Design review of the part built by this model. Coordinates are the model's own, in mm. Face numbers are marked on the shaded views. A direction names the side the tool comes from. Round coordinates to 2 decimals unless told otherwise and drop trailing zeros. Loops run counter-clockwise (first coordinate to the right, second up) from the corner with the lowest first, then second, coordinate; pieces in that order, holes last. Notation, with made-up numbers: (49, 31.5) - (55, 31.5) arc R26 cw to (55, 57.5) - close; hole circle Ø6 at (-40, 77). An arc over 180 degrees is marked (long way). Return JSON: item names as keys, results as strings. Group by question number.
(1) We need section C-C, the plane x = 25.5. Write out the cut boundary in (y, z), and give its area (3 significant figures).
(2) For the marked faces 1 and 2, list the 3-axis set-ups (+Z, -Z, +X, -X, +Y, -Y) from which the entire face can be reached by the end or side of a thin tool; tool diameter is ignored.
(3) The part is to be moulded in two halves that separate along X. For the marked faces 3, 4 and 5, say which applies: pulls with the +X half, pulls with the -X half, needs draft (parallel to the pull), parting line crosses it, or undercut.
(4) Clearance check with flat-ended pins moving along their axes: pin 1 (3.5 mm diameter, centred on x = 16, z = 26, fed in from -Y); pin 2 (1.5 mm diameter, centred on x = 14, y = 4.5, fed in from +Z); pin 3 (2.5 mm diameter, centred on x = 25.5, y = 6.5, fed in from -Z). State where each tip first meets the part, or that it passes through.
(5) We need section D-D, the plane z = 26. Give the number of separate pieces and of enclosed holes in the cut face, and give its area (3 significant figures).
(6) We need section A-A, the plane z = 51.5. Write out the cut boundary in (x, y).
(7) Wall thickness on L1, parallel to Z at x = 29.75, y = 6.5; L2, parallel to Y at x = 1.7, z = 26; L3, parallel to X at y = 6.5, z = 62.4: over which ranges is each line inside the solid? List them lowest first. Write a range as [from, to].
(8) We need section B-B, the plane y = 11.5. Write out the cut boundary in (x, z).
from build123d import *

# Parameters (mm, degrees)
F1_DEPTH  = 13
F2_R      = 1.5
F3_DEPTH  = 12
F4_R      = 1.5
F5_DEPTH  = 32.001
F6_DEPTH  = 32.001
F7_R      = 2
F8_DEPTH  = 6
F9_R      = 1
F10_DEPTH = 32.001
F11_R     = 1
F12_DEPTH = 5
F13_R     = 1
F14_DEPTH = 3.001
F15_R     = 1
F16_DEPTH = 3.001
F17_R     = 0.75
F18_DEPTH = 5.7019619943


with BuildPart() as f1:
    # F0 (on Front) → F1 (new body)
    with BuildSketch(Plane.XZ):
        Polygon((0, 64), (0, 0), (32, 0), (32, 64), (24, 64), (24, 37), (8, 37), (8, 64), align=None)
    extrude(amount=-F1_DEPTH)

    # F2 (on face) → F3 (cut)
    with BuildSketch(Plane(origin=(0, 0, 0), x_dir=(1, 0, 0), z_dir=(0, 0, -1))):
        with Locations((6.5, -6.5)):
            Circle(F2_R)
        with Locations((25.5, -6.5)):
            Circle(F2_R)
    extrude(amount=-F3_DEPTH, mode=Mode.SUBTRACT)

    # F4 (on face) → F5 (cut, through all)
    with BuildSketch(Plane.YZ.offset(32)):
        with Locations((6.5, 57)):
            Circle(F4_R)
    extrude(amount=-F5_DEPTH, mode=Mode.SUBTRACT)

    # F4 (on face) → F6 (cut, through all)
    with BuildSketch(Plane.YZ.offset(32)):
        with Locations((6.5, 16)):
            Circle(F4_R)
    extrude(amount=-F6_DEPTH, mode=Mode.SUBTRACT)

    # F7 (on face) → F8 (cut)
    with BuildSketch(Plane.XZ):
        with Locations((16, 26)):
            Circle(F7_R)
    extrude(amount=-F8_DEPTH, mode=Mode.SUBTRACT)

    # F9 (on face) → F10 (cut, through all)
    with BuildSketch(Plane(origin=(0, 0, 0), x_dir=(0, -1, 0), z_dir=(-1, 0, 0))):
        with Locations((-3.5, 26)):
            Circle(F9_R)
    extrude(amount=-F10_DEPTH, mode=Mode.SUBTRACT)

    # F11 (on face) → F12 (cut)
    with BuildSketch(Plane(origin=(0, 13, 0), x_dir=(-1, 0, 0), z_dir=(0, 1, 0))):
        with Locations((-29, 26)):
            Circle(F11_R)
        with Locations((-3, 26)):
            Circle(F11_R)
    extrude(amount=-F12_DEPTH, mode=Mode.SUBTRACT)

    # F13 (on face) → F14 (cut, through all)
    with BuildSketch(Plane(origin=(0, 0, 0), x_dir=(0, -1, 0), z_dir=(-1, 0, 0))):
        with Locations((-9.5, 26)):
            Circle(F13_R)
    extrude(amount=-F14_DEPTH, mode=Mode.SUBTRACT)

    # F15 (on face) → F16 (cut, through all)
    with BuildSketch(Plane.YZ.offset(32)):
        with Locations((9.5, 26)):
            Circle(F15_R)
    extrude(amount=-F16_DEPTH, mode=Mode.SUBTRACT)

    # F17 (on face) → F18 (cut, through all)
    with BuildSketch(Plane.XY.offset(64)):
        with Locations((4, 6.5)):
            Circle(F17_R)
        with Locations((28, 6.5)):
            Circle(F17_R)
    extrude(amount=-F18_DEPTH, mode=Mode.SUBTRACT)


solid = f1.part
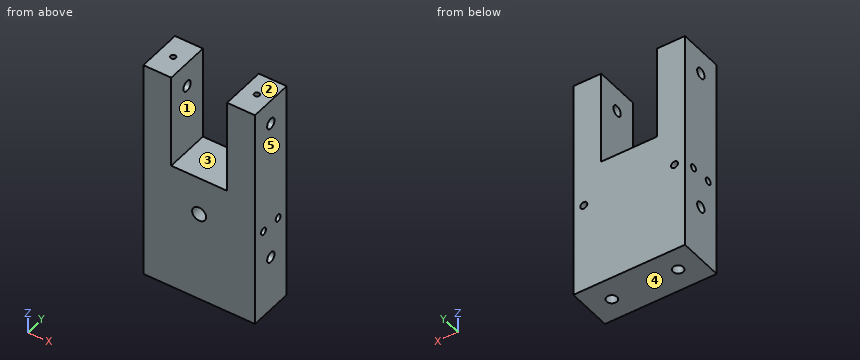
Solutions:
{
 "1": {"outline": "(0, 0) - (5, 0) - (5, 12) - (8, 12) - (8, 0) - (13, 0) - (13, 64) - (0, 64) - close; hole circle Ø2 at (3.5, 26); hole circle Ø3 at (6.5, 16); hole circle Ø3 at (6.5, 57)", "area": "779 mm^2"},
 "2": {"face 1": "+Z, +Y, -Y", "face 2": "+Z, +X, -X, +Y, -Y"},
 "3": {"face 3": "undercut", "face 4": "needs draft", "face 5": "pulls with the +X half"},
 "4": {"pin 1": "y = 6", "pin 2": "z = 37", "pin 3": "z = 12"},
 "5": {"separate pieces": "5", "enclosed holes": "0", "area": "308 mm^2"},
 "6": {"outline": "(0, 0) - (8, 0) - (8, 13) - (0, 13) - close; (24, 0) - (32, 0) - (32, 13) - (24, 13) - close"},
 "7": {"L1": "[0, 14.5], [17.5, 55.5], [58.5, 64]", "L2": "[0, 2.5], [4.5, 8.5], [10.5, 13]", "L3": "[0, 3.25], [4.75, 8], [24, 27.25], [28.75, 32]"},
 "8": {"outline": "(0, 0) - (32, 0) - (32, 64) - (24, 64) - (24, 37) - (8, 37) - (8, 64) - (0, 64) - close; hole circle Ø2 at (3, 26); hole circle Ø2 at (29, 26)"}
}
